from build123d import *

# Parameters (mm, degrees)
F0_R     = 63.9996610984
F0_R_2   = 52.8119822493
F1_DEPTH = 20
F2_R     = 21.3194523792
F3_DEPTH = 20
F5_W     = 44.8123216629
F5_H     = 14.4665837288
F4_W     = 16.3650214672
F4_H     = 105.4660975933
F6_DEPTH = 20


with BuildPart() as f1:
    # F0 (on Top) → F1 (new body)
    with BuildSketch(Plane.XY):
        Circle(F0_R)
        Circle(F0_R_2, mode=Mode.SUBTRACT)
    extrude(amount=F1_DEPTH)



with BuildPart() as f3:
    # F2 (on Top) → F3 (new body)
    with BuildSketch(Plane.XY):
        Circle(F2_R)
    extrude(amount=F3_DEPTH)


with BuildPart() as f1_1:
    add(f1.part)

    add(f3.part)  # F6 merges F3
    # F5 (on face) + F4 (on Top) → F6 (join)
    with BuildSketch(Plane.XY):
        with Locations((-30.5886715651, 0)):
            Rectangle(F5_W, F5_H)
        with Locations((30.5886715651, 0)):
            Rectangle(F5_W, F5_H)
    with BuildSketch(Plane.XY):
        Rectangle(F4_W, F4_H)
    extrude(amount=F6_DEPTH)


solid = f1_1.part
Build history of the part. All positions in model axes, mm. A direction names the side the tool comes from. Give positions to 0.01 mm unless a question says otherwise; leave off trailing zeros. Order: outer loops, then holes, each group sorted by start corner. A loop starts at its lowest first (then second) coordinate and runs counter-clockwise, first axis right, second up. Notation, with made-up numbers: M -32,-3 L -1,-3 A36 ccw -1,32 Z; hole C -33,74.5 d8. An arc over 180 degrees is marked long. Use one line per item in the form item = value.
Q1. Slice it at C-C, the plane y = 12. Write the cut outline in (x, z).
Conclusion:
outline = M -62.86,0 L -51.43,0 L -51.43,20 L -62.86,20 Z; M -17.62,0 L 17.62,0 L 17.62,20 L -17.62,20 Z; M 51.43,0 L 62.86,0 L 62.86,20 L 51.43,20 Z
Q2. Which spindle directions (+Z, -Z, +X, -X, +Y, -Y) get a long thin tool onto all of the face, cutting with end or side? Do faces 4 (the flat face through (-1, 1, 20)), 5 (the flat face through (8.183, 36, 10)). Say none if no direction does.
Conclusion:
face_4 = +Z, +X, -X, +Y, -Y
face_5 = +Z, -Z
Q3. Wall check: probe 1 along Y at (x, z) = (34.5, 11.5); probe 2 along X at (y, z) = (27, 13.25); probe 3 along Y at (x, z) = (-28, 14.75). Give the ranges that are in metal, low to high.
Conclusion:
probe_1 = -53.9 to -39.99, -7.23 to 7.23, 39.99 to 53.9
probe_2 = -58.03 to -45.39, -8.18 to 8.18, 45.39 to 58.03
probe_3 = -57.55 to -44.78, -7.23 to 7.23, 44.78 to 57.55
Q4. Slice it at D-D, the plane y = -56. Write the cut outline in (x, z), and give its area (3 significant figures).
Conclusion:
outline = M -30.98,0 L 30.98,0 L 30.98,20 L -30.98,20 Z
area = 1,240 mm2
Q5. Pull direction X, two halves, no side cores. Call faces 1 (the cylindrical face through (-63.938, 2.814, 9.86)), 2 (the flat face through (-8.183, -36, 10)), 3 (the flat face through (-1, 1, 0)): released by +X, released by -X, zero draft, split by the parting line, or undercut.
Conclusion:
face_1 = split by the parting line
face_2 = undercut
face_3 = zero draft
Q6. Slice it at B-B, the plane x = 37.5. Write the cut outline in (y, z).
Conclusion:
outline = M -51.86,0 L -37.19,0 L -37.19,20 L -51.86,20 Z; M -7.23,0 L 7.23,0 L 7.23,20 L -7.23,20 Z; M 37.19,0 L 51.86,0 L 51.86,20 L 37.19,20 Z
Q7. Pin check, flat tips, straight feed: P1, Ø10, axis at x = 32.5, z = 12, coming from the +Y side; P2, Ø6, axis at x = -10.5, y = 39, coming from the +Z side; P3, Ø4, axis at x = 45.5, z = 10, coming from the +Y side; P4, Ø10, axis at x = 11.5, z = 17, coming from the -Y side. Stop position of each tip, or through.
Conclusion:
P1 = 57.79
P2 = 20
P3 = 46.94
P4 = -63.67
Q8. Slice it at A-A, the plane z = 1.5. Write the cut outline in (x, y), and give its area (3 significant figures).
Conclusion:
outline = C 0,0 d128; hole M -52.31,-7.23 A52.81 ccw -8.18,-52.17 L -8.18,-19.69 A21.32 cw -20.05,-7.23 Z; hole M -52.31,7.23 L -20.05,7.23 A21.32 cw -8.18,19.69 L -8.18,52.17 A52.81 ccw Z; hole M -2.89,-52.73 A52.81 ccw 2.89,-52.73 Z; hole M -2.89,52.73 L 2.89,52.73 A52.81 ccw Z; hole M 8.18,-52.17 A52.81 ccw 52.31,-7.23 L 20.05,-7.23 A21.32 cw 8.18,-19.69 Z; hole M 8.18,19.69 A21.32 cw 20.05,7.23 L 52.31,7.23 A52.81 ccw 8.18,52.17 Z
area = 7,490 mm2
